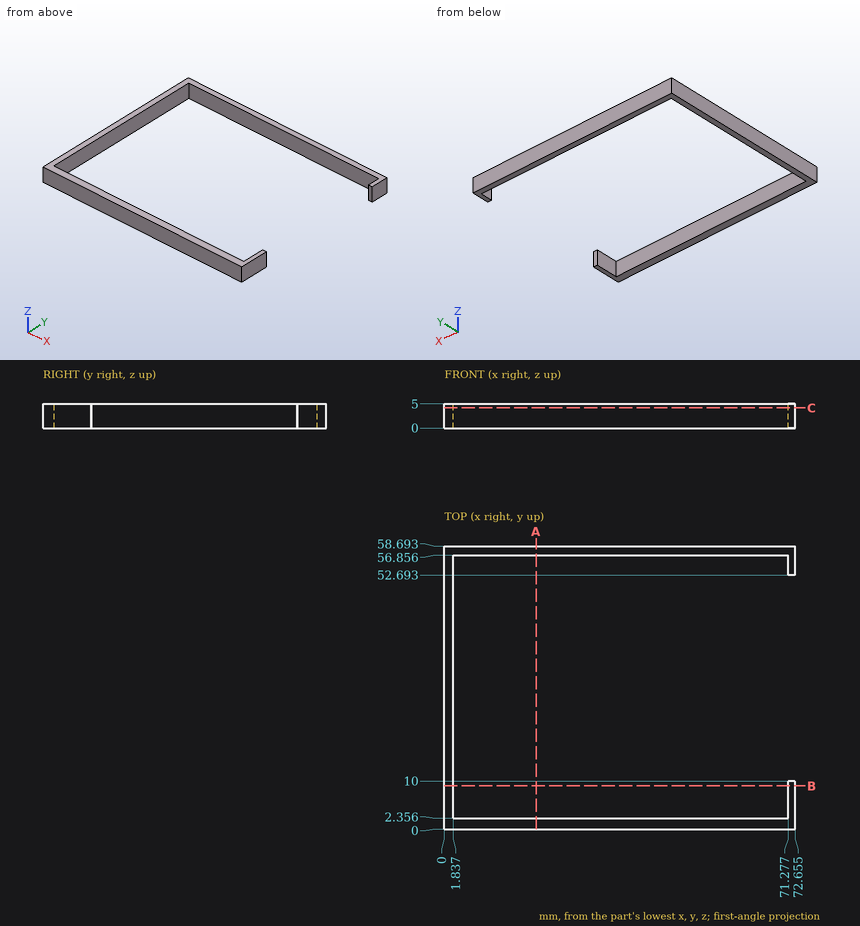
Part print with two shaded views. Sizes in mm from the minimum x, y, z corner. Coordinates: 2 decimals unless noted, no trailing zeros. Order: outer loops, then holes, each group sorted by start corner. A loop starts at its lowest first (then second) coordinate and runs counter-clockwise, first axis right, second up.
(1) Saw through at C-C, the plane z = 4.2. Write the cut outline in (x, y) (1 decimal), and give its area (3 significant figures).
Solution:
outline: (0, 0) - (72.7, 0) - (72.7, 10) - (71.3, 10) - (71.3, 2.4) - (1.8, 2.4) - (1.8, 56.9) - (71.3, 56.9) - (71.3, 52.7) - (72.7, 52.7) - (72.7, 58.7) - (0, 58.7) - close
area: 421 mm2
(2) Saw through at A-A, the plane x = 19. Write the cut outline in (y, z).
Solution:
outline: (0, 0) - (2.36, 0) - (2.36, 5) - (0, 5) - close; (56.86, 0) - (58.69, 0) - (58.69, 5) - (56.86, 5) - close
(3) Saw through at B-B, the plane y = 9. Write the cut outline in (x, z) (1 decimal).
Solution:
outline: (0, 0) - (1.8, 0) - (1.8, 5) - (0, 5) - close; (71.3, 0) - (72.7, 0) - (72.7, 5) - (71.3, 5) - close
(4) Pin check, flat tip, straight feed: pin 1 Ø1.5 at (y, z) = (24.5, 3.5) entering from +X. Stop position of the tip, or through.
Solution:
pin 1: stops at x = 1.84
(5) Drill centre lines: L1, parallel to Y at x = 43.5, z = 1.7; L2, parallel to X at y = 4.5, z = 1.8 (1 decimal); L3, parallel to X at y = 29, z = 4.65. Where is each one in solid material? Low to high.
Solution:
L1: y = 0 to 2.36, 56.86 to 58.69
L2: x = 0 to 1.8, 71.3 to 72.7
L3: x = 0 to 1.84
